Build history of the part. All positions in model axes, mm. Coordinates: 2 decimals unless noted, no trailing zeros. Write each loop counter-clockwise with the first axis right and the second up, starting at its lowest first coordinate (ties: lowest second). Pieces come first, ordered by that corner, then holes.
```python
from build123d import *

# Parameters (mm, degrees)
CYLINDER007_R     = 1.6
CYLINDER007_DEPTH = 10
CYLINDER006_R     = 1.6
CYLINDER006_DEPTH = 10
CYLINDER005_R     = 1.6
CYLINDER005_DEPTH = 10
CYLINDER004_R     = 1.6
CYLINDER004_DEPTH = 10
BOX001_W          = 104
BOX001_H          = 62
BOX001_DEPTH      = 4


with BuildPart() as mount_point003:
    # Cylinder007 → Cylinder007 (new body)
    with BuildSketch(Plane(origin=(-3.1, 58.9, 0), x_dir=(1, 0, 0), z_dir=(0, 0, 1))):
        Circle(CYLINDER007_R)
    extrude(amount=CYLINDER007_DEPTH)


with BuildPart() as mount_point002:
    # Cylinder006 → Cylinder006 (new body)
    with BuildSketch(Plane(origin=(-100.9, 58.9, 0), x_dir=(1, 0, 0), z_dir=(0, 0, 1))):
        Circle(CYLINDER006_R)
    extrude(amount=CYLINDER006_DEPTH)


with BuildPart() as mount_point001:
    # Cylinder005 → Cylinder005 (new body)
    with BuildSketch(Plane(origin=(-100.9, 3.1, 0), x_dir=(1, 0, 0), z_dir=(0, 0, 1))):
        Circle(CYLINDER005_R)
    extrude(amount=CYLINDER005_DEPTH)


with BuildPart() as mount_point:
    # Cylinder004 → Cylinder004 (new body)
    with BuildSketch(Plane(origin=(-2.6, 3.1, 0), x_dir=(1, 0, 0), z_dir=(0, 0, 1))):
        Circle(CYLINDER004_R)
    extrude(amount=CYLINDER004_DEPTH)


with BuildPart() as standard_platform:
    # Box001 → Box001 (new body)
    with BuildSketch(Plane(origin=(-104, 0, 0), x_dir=(1, 0, 0), z_dir=(0, 0, 1))):
        with Locations((52, 31)):
            Rectangle(BOX001_W, BOX001_H)
    extrude(amount=BOX001_DEPTH)

    # Cut005: cut Mount Point
    add(mount_point.part, mode=Mode.SUBTRACT)

    # Cut006: cut Mount Point001
    add(mount_point001.part, mode=Mode.SUBTRACT)

    # Cut007: cut Mount Point002
    add(mount_point002.part, mode=Mode.SUBTRACT)

    # Cut008: cut Mount Point003
    add(mount_point003.part, mode=Mode.SUBTRACT)


solid = standard_platform.part
```
1. Probe line 1 along Y through (x, z) = (-100.9, 2.35); line 2 along X through (y, z) = (58.9, 3.2); line 3 along X through (y, z) = (3.1, 3.05). List the from-to ranges inside material, lowest first.
Computed values:
line 1: y = 0 to 1.5, 4.7 to 57.3, 60.5 to 62
line 2: x = -104 to -102.5, -99.3 to -4.7, -1.5 to 0
line 3: x = -104 to -102.5, -99.3 to -4.2, -1 to 0
2. Saw through at B-B on y = 58.9. List the corners of the cut face in (x, z).
Computed values:
outline: (-104, 0) - (-102.5, 0) - (-102.5, 4) - (-104, 4) - close; (-99.3, 0) - (-4.7, 0) - (-4.7, 4) - (-99.3, 4) - close; (-1.5, 0) - (0, 0) - (0, 4) - (-1.5, 4) - close
3. Saw through at A-A on x = -100.9. List the corners of the cut face in (y, z).
Computed values:
outline: (0, 0) - (1.5, 0) - (1.5, 4) - (0, 4) - close; (4.7, 0) - (57.3, 0) - (57.3, 4) - (4.7, 4) - close; (60.5, 0) - (62, 0) - (62, 4) - (60.5, 4) - close
4. Mould opens along X. For faces 1 (the face through (-104, 31, 2)), 2 (the face through (-53, 62, 2)), 3 (the face through (-1.074, 3.581, 1.972)) say: +X half, -X half, draft (parallel to the pull), parting line (faces both ways), or undercut.
Computed values:
face 1: -X half
face 2: draft
face 3: undercut
